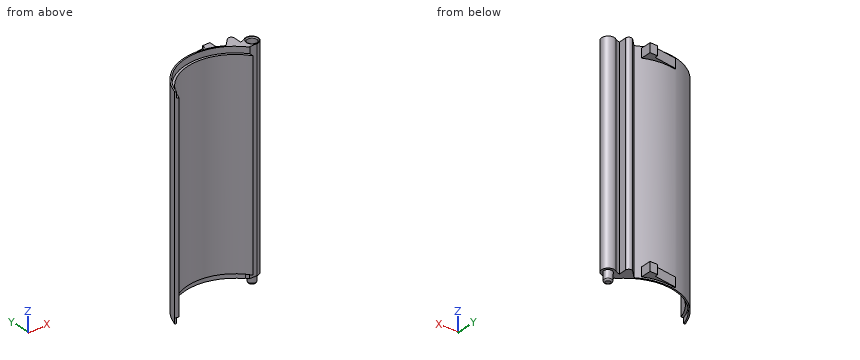
from build123d import *

# Parameters (mm, degrees)
BOSS_EXTRU_1_DEPTH      = 1.8
BOSS_EXTRU_2_DEPTH      = 67.6
ESQUISSE3_R             = 1.35
BOSS_EXTRU_3_DEPTH      = 3
BOSS_EXTRU_3_DRAFT      = -2
BOSS_EXTRU_4_DEPTH      = 69.4
CONG_1_R                = 5
ESQUISSE5_R             = 1.55
ENL_V_MAT_EXTRU_1_DEPTH = 20
BOSS_EXTRU_5_START      = 0.486262707
BOSS_EXTRU_5_DEPTH      = 3
ENL_V_START             = -2
ENL_V_MAT_EXTRU_2_DEPTH = 2
ENL_V_MAT_EXTRU_3_DEPTH = 83.186412318
BOSS_EXTRU_6_DEPTH      = 69.4
CONG_2_R                = 1
CONG_3_R                = 0.3
CONG_4_R                = 0.5


# Read off the part's stored shape, not the designer's step: Boss.-Extru.5
with BuildPart() as part:
    # Esquisse1 → Boss.-Extru.1 (new body)
    with BuildSketch(Plane.XY):
        with BuildLine():
            Line((-33.169498422, 7.22242532), (-33.600967303, 7.350232225))
            ThreePointArc((-33.600967303, 7.350232225), (-21.461995756, 18.851787613), (-5.439284285, 14.065022141))
            Line((-5.439284285, 14.065022141), (-5.439284285, 13.398595658))
            ThreePointArc((-5.439284285, 13.398595658), (-21.121374045, 18.468530159), (-33.169498422, 7.22242532))
        make_face()
    extrude(amount=BOSS_EXTRU_1_DEPTH)

    # Esquisse2 → Boss.-Extru.2 (add)
    with BuildSketch(Plane.XY.offset(1.8)):
        with BuildLine():
            Line((-33.600967303, 7.350232225), (-32.450383621, 7.009413812))
            ThreePointArc((-32.450383621, 7.009413812), (-19.947199013, 17.926685666), (-4.739284285, 11.275687265))
            Line((-4.739284285, 11.275687265), (-4.739284285, 13.274091553))
            ThreePointArc((-4.739284285, 13.274091553), (-5.083029835, 13.675092245), (-5.439284285, 14.065022141))
            ThreePointArc((-5.439284285, 14.065022141), (-21.461995756, 18.851787613), (-33.600967303, 7.350232225))
        make_face()
    extrude(amount=BOSS_EXTRU_2_DEPTH)



with BuildPart() as body_2:
    # Esquisse3 → Boss.-Extru.3 (with draft: the straight prism first)
    with BuildSketch(Plane.XY):
        with Locations((-2.219642143, 14.857175969)):
            Circle(ESQUISSE3_R)
    extrude(amount=-BOSS_EXTRU_3_DEPTH)
    # Boss.-Extru.3: the draft: its side faces are tilted about the plane it starts from
    boss_extru_3_sides = [body_2.faces().sort_by_distance(p)[0] for p in [
        (-3.569642143, 14.857175969, -1.5),
    ]]
    draft(boss_extru_3_sides, Plane.XY, BOSS_EXTRU_3_DRAFT)


with BuildPart() as part_1:
    add(part.part)

    add(body_2.part)  # Boss.-Extru.4 merges body 2
    # Esquisse4 → Boss.-Extru.4 (add)
    with BuildSketch(Plane.XY):
        with BuildLine():
            Line((-2.233779809, 12.757223558), (-4.739284285, 12.774091553))
            Line((-4.739284285, 12.774091553), (-6.149439768, 14.774091553))
            Line((-6.149439768, 14.774091553), (-3.378858565, 16.608237729))
            ThreePointArc((-3.378858565, 16.608237729), (-0.206741875, 15.455701249), (-2.233779809, 12.757223558))
        make_face()
    extrude(amount=BOSS_EXTRU_4_DEPTH)

    # Congé1
    cong_1_edges = [part_1.edges().sort_by_distance(p)[0] for p in [
        (-6.149439768, 14.774091553, 34.7),
    ]]
    fillet(cong_1_edges, radius=CONG_1_R)

    # Esquisse5 → Enlèv. mat.-Extru.1 (cut)
    with BuildSketch(Plane.XY.offset(69.4)):
        with Locations((-2.219642143, 14.857175969)):
            Circle(ESQUISSE5_R)
    extrude(amount=-ENL_V_MAT_EXTRU_1_DEPTH, mode=Mode.SUBTRACT)

    # Boss.-Extru.5 outline → Boss.-Extru.5 (add)
    with BuildSketch(Plane.XY.offset(BOSS_EXTRU_5_START)):
        with BuildLine():
            Line((-10.832608102, 17.879553752), (-10.832608102, 21.307175969))
            Line((-10.832608102, 21.307175969), (-20.832608102, 21.307175969))
            Line((-20.832608102, 21.307175969), (-20.832608102, 18.989084153))
            ThreePointArc((-20.832608102, 18.989084153), (-15.747062959, 19.205322101), (-10.832608102, 17.879553752))
        make_face()
    boss_extru_5 = extrude(amount=BOSS_EXTRU_5_DEPTH)

    # Symétrie1: Boss.-Extru.5 across plane
    add(boss_extru_5.mirror(Plane.XY.offset(34.7)))

    # Esquisse7 → Enlèv. mat.-Extru.2 (cut)
    with BuildSketch(Plane.XY.offset(69.4).offset(ENL_V_START)):
        with BuildLine():
            Line((-32.450383621, 7.009413812), (-33.169498422, 7.22242532))
            ThreePointArc((-33.169498422, 7.22242532), (-20.584304116, 18.578673161), (-4.739284285, 12.554818307))
            Line((-4.739284285, 12.554818307), (-4.739284285, 11.275687265))
            ThreePointArc((-4.739284285, 11.275687265), (-19.947199013, 17.926685666), (-32.450383621, 7.009413812))
        make_face()
    extrude(amount=ENL_V_MAT_EXTRU_2_DEPTH, mode=Mode.SUBTRACT)

    # Esquisse9 → Enlèv. mat.-Extru.3 (cut, through all)
    with BuildSketch(Plane.XY.offset(68.913737293)):
        Polygon((-20.832608102, 19.307175969), (-13.332608102, 20.294569701), (-13.332608102, 21.307175969), (-20.832608102, 21.307175969), align=None)
    extrude(amount=-ENL_V_MAT_EXTRU_3_DEPTH, mode=Mode.SUBTRACT)

    # Esquisse10 → Boss.-Extru.6 (add)
    with BuildSketch(Plane.XY.offset(69.4)):
        Polygon((-5.019642143, 15.993667324), (-5.019642143, 20.993667324), (-9.052568259, 16.960741208), (-4.646335714, 14.274994024), align=None)
    extrude(amount=-BOSS_EXTRU_6_DEPTH)

    # Congé2
    cong_2_edges = [part_1.edges().sort_by_distance(p)[0] for p in [
        (-5.019642143, 20.993667324, 34.7),
    ]]
    fillet(cong_2_edges, radius=CONG_2_R)

    # Congé3
    cong_3_edges = [part_1.edges().sort_by_distance(p)[0] for p in [
        (-3.769642143, 14.857175969, 69.4),
    ]]
    fillet(cong_3_edges, radius=CONG_3_R)

    # Congé4
    cong_4_edges = [part_1.edges().sort_by_distance(p)[0] for p in [
        (-3.464879834, 14.857175969, -3),
    ]]
    fillet(cong_4_edges, radius=CONG_4_R)


solid = part_1.part
Geometry check sheet. Reference: the model listing, model coordinates, mm. Give positions to 0.01 mm unless a question says otherwise; leave off trailing zeros. Loops run counter-clockwise (first coordinate to the right, second up) from the corner with the lowest first, then second, coordinate; pieces in that order, holes last.
(1) Section check A-A on x = -20. Record the cut outline in (y, z), then the cut area to 3 significant figures.
From the geometry:
outline: (17.92, 1.8) - (18.68, 1.8) - (18.68, 0) - (19.13, 0) - (19.13, 0.49) - (19.42, 0.49) - (19.42, 3.49) - (19.13, 3.49) - (19.13, 65.91) - (19.42, 65.91) - (19.42, 68.91) - (19.13, 68.91) - (19.13, 69.4) - (18.68, 69.4) - (18.68, 67.4) - (17.92, 67.4) - close
area: 83.1 mm2
(2) Depth check by flat-ended pin: pin 1 Ø0.5 at (y, z) = (21, 2.5) entering from -X; pin 2 Ø6 at (x, z) = (-15, 31.5) entering from +Y; pin 3 Ø2.5 at (x, y) = (-16.5, 19) entering from -Z. Enter the tip coordinate at first touch or a pass-through.
From the geometry:
pin 1: stops at x = -13.33
pin 2: stops at y = 19.31
pin 3: stops at z = 0
(3) Section check D-D on x = -16.5. Record the cut outline in (y, z).
From the geometry:
outline: (18.07, 1.8) - (18.82, 1.8) - (18.82, 0) - (19.27, 0) - (19.27, 0.49) - (19.88, 0.49) - (19.88, 3.49) - (19.27, 3.49) - (19.27, 65.91) - (19.88, 65.91) - (19.88, 68.91) - (19.27, 68.91) - (19.27, 69.4) - (18.82, 69.4) - (18.82, 67.4) - (18.07, 67.4) - close
(4) Section check B-B on z = 51. Count the separate pieces of the cut face and the enclosed holes in it, then the cut area to 3 significant figures.
From the geometry:
separate pieces: 1
enclosed holes: 2
area: 65.2 mm2
(5) Section check C-C on x = -10. Record the cut outline in (y, z).
From the geometry:
outline: (16.12, 1.8) - (16.98, 1.8) - (16.98, 0) - (17.48, 0) - (17.48, 69.4) - (16.98, 69.4) - (16.98, 67.4) - (16.12, 67.4) - close
(6) Thickness scan on L1, parallel to Z at x = -17.5, y = 19.5; L2, parallel to Y at x = -4.5, z = 19.5; L3, parallel to X at y = 14.25, z = 30. Record the ranges inside material, lowest first.
From the geometry:
L1: z = 0.49 to 3.49, 65.91 to 68.91
L2: y = 12.77 to 16.12
L3: x = -29.56 to -27.82, -7.36 to -0.21
